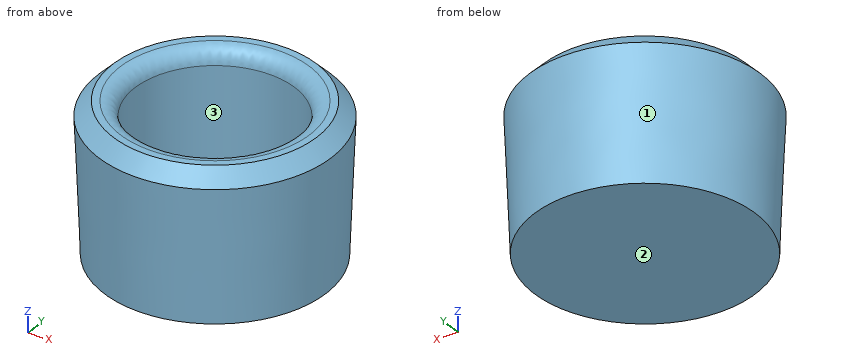
```python
from build123d import *

# Parameters (mm, degrees)
F2_R    = 5.08
F3_SIZE = 5.08


with BuildPart() as f1:
    # F0 (on Right) → F1 (revolve)
    with BuildSketch(Plane.YZ):
        Polygon((-46.0525572707, -5.5384264588), (-46.0525572707, 41.3120244363), (-58.5525572707, 41.4615735412), (-56.5525572707, -8.5384264588), (-19.0525572707, -8.5384264588), (-19.0525572707, -5.5384264588), align=None)
    revolve(axis=Axis((0, -19.0525572707, -7.0384264588), (0, 0, -1)))

    # F2
    f2_edges = [f1.edges().sort_by_distance(p)[0] for p in [
        (0, 7.947443, 41.312024),
    ]]
    fillet(f2_edges, radius=F2_R)

    # F3
    f3_edges = [f1.edges().sort_by_distance(p)[0] for p in [
        (0, 20.447443, 41.461574),
    ]]
    chamfer(f3_edges, length=F3_SIZE)


solid = f1.part
```
Build history of the part. All positions in model axes, mm. Face numbers are marked on the shaded views. Coordinates: 2 decimals unless noted, no trailing zeros. Order: outer loops, then holes, each group sorted by start corner. A loop starts at its lowest first (then second) coordinate and runs counter-clockwise, first axis right, second up. Notation, with made-up numbers: M 28,-18 L 41,-18 A23 ccw 41,-5 Z; hole C 17.25,72 d1. An arc over 180 degrees is marked long. One line per question, with ' | ' between items. Start each with the question number.
1. Flat gauge pins, fed straight in: P1, Ø1.5, axis at x = -6, z = 31, coming from the +Y side; P2, Ø12, axis at y = -44, z = 11.5, coming from the -X side; P3, Ø2, axis at y = 7, z = 31, coming from the -X side. Where does each tip first touch, or does it go through?
2. Mould opens along Y. For the marked faces 1, 2 and 3 say: +Y half, -Y half, draft (parallel to the pull), parting line (faces both ways), or undercut.
3. Cut at B-B (z = -1). Write the cut outline in (x, y), plus the area to 3 significant figures.
4. Wall check: line 1 along Z through (x, y) = (-18.5, -35); line 2 along Z through (x, y) = (25.5, 2); line 3 along Y through (x, z) = (0, 5). Give the ranges that are in metal, low to high. Write a range as [from, to].
5. Cut at A-A (z = 21). Write the cut outline in (x, y), plus the area to 3 significant figures.
The answers:
1) P1: stops at y = 19.68 | P2: stops at x = -33.3 | P3: stops at x = -30
2) face 1: parting line | face 2: draft | face 3: undercut
3) outline: C 0,-19.05 d75.6; hole C 0,-19.05 d54 | area: 2,200 mm2
4) line 1: z = [-8.54, -5.54] | line 2: z = [-8.54, 41.38] | line 3: y = [-57.09, -46.05], [7.95, 18.99]
5) outline: C 0,-19.05 d77.36; hole C 0,-19.05 d54 | area: 2,410 mm2
